Input: part model. Units: mm. Frame: model coordinates. A direction names the side the tool comes from. Coordinates: 2 decimals unless noted, no trailing zeros. Order: outer loops, then holes, each group sorted by start corner. A loop starts at its lowest first (then second) coordinate and runs counter-clockwise, first axis right, second up. Notation, with made-up numbers: (-38, 56) -> (6, 56) arc R22 cw to (6, 85) -> close; hole circle Ø10 at (3, 84.25). An arc over 180 degrees is marked (long way). One line per question, with ' | ' between items.
Autodesk Inventor part; units mm, degrees
ref_plane "YZ Plane" through (0, 0, 0) normal (1, 0, 0) x (0, 1, 0)
ref_plane "XZ Plane" through (0, 0, 0) normal (0, 1, 0) x (-1, 0, 0)
ref_plane "XY Plane" through (0, 0, 0) normal (0, 0, 1) x (1, 0, 0)
sketch "Эскиз1" plane through (0, 0, 0) normal (0, 1, 0) x (-1, 0, 0)
  line L0 (0, 0) -> (4, 0)
  line L1 (4, 0) -> (4, -23.9397)
  line L2 (4, -23.9397) -> (0, -23.9397)
  line L3 (0, -23.9397) -> (0, 0)
  line L4 (0, -23.9397) -> (11.75, -23.9397)
  line L5 (11.75, -23.9397) -> (11.75, -19.9397)
  line L6 (11.75, -19.9397) -> (0, -19.9397)
  line L7 (0, -19.9397) -> (0, -23.9397)
  line L8 (11.75, -19.9397) -> (7.75, -19.9397)
  line L9 (7.75, -19.9397) -> (7.75, -29.9397)
  line L10 (7.75, -29.9397) -> (11.75, -29.9397)
  line L11 (11.75, -29.9397) -> (11.75, -19.9397)
  line L12 (11.75, -23.9397) -> (4, -19.9397)
  line L13 (0, -19.9397) -> (7.75, -23.9397)
  point P0 (3, -20.536)
  point P1 (0, -19.9397)
  dimension "d10" = 4
  dimension "d11" = 11.75
  dimension "d36" = 29.9397
  dimension "d55" = 10
extrude "Выдавливание1" add sketch "Эскиз1" along normal blind 5
fillet "Сопряжение2" radius 3.855 4 edges at (-4, 2.5, -19.9397) (-11.75, 2.5, -19.9397) (0, 2.5, -23.9397) (-7.75, 2.5, -23.9397)
sketch "Эскиз7" plane through (-11.75, 0, -29.9397) normal (-1, 0, 0) x (0, 0, 1)
  line L0 (0, 0) -> (0, 5)
  circle A0 centre (0, 2.5) radius 2.525
  circle A1 centre (0, 2.5) radius 3.525
  point P0 (29.9397, 0)
  point P1 (0, 4.975)
  point P2 (0, 0.025)
  dimension "d37" = 5.05
  dimension "d38" = 7.05
extrude "Выдавливание5" add sketch "Эскиз7" against normal up to surface (4 mm away) contours A0 | A1
extrude "Выдавливание8" cut sketch "Эскиз7" against normal through all contours A0
sketch "Эскиз8" plane through (-4, 0, 0) normal (-1, 0, 0) x (0, 0, 1)
  line L0 (0, 0) -> (0, 5)
  circle A0 centre (0, 2.5) radius 2.525
  circle A1 centre (0, 2.5) radius 3.525
  point P0 (0, 4.975)
  point P1 (0, 0.025)
  dimension "d41" = 5.05
  dimension "d42" = 7.05
extrude "Выдавливание6" add sketch "Эскиз8" against normal up to surface (4 mm away)
extrude "Выдавливание7" cut sketch "Эскиз8" against normal through all contours A0
sketch "Эскиз9" plane through (-4, 0, -20.0847) normal (1, 0, 0) x (0, 0, -1)
  circle A0 centre (-20.0847, 2.5) radius 2.525
  circle A1 centre (-20.0847, 2.5) radius 4.025
  arc A2 (-17.5996, 5) -> (-17.5996, 0) centre (-20.0847, 2.5) ccw
  point P0 (-20.0847, 0)
  point P1 (-20.0847, 4.975)
  point P2 (-20.0847, 0.025)
  point P3 (-19.7302, 5)
  point P4 (-19.7302, 0)
  dimension "d49" = 0.5
extrude "Выдавливание9" cut sketch "Эскиз9" along normal blind 2.25 contours A0 | A1
sketch "Эскиз10" plane through (0, 0, -16.0847) normal (-1, 0, 0) x (0, 0, 1)
  arc A0 (13.5996, 0) -> (13.5996, 5) centre (16.0847, 2.5) ccw
  circle A1 centre (16.0847, 2.5) radius 3.525
  circle A2 centre (16.0847, 2.5) radius 2.525
  point P0 (12.3578, 0)
  point P1 (12.3578, 5)
  point P2 (13.5996, 5)
  point P3 (13.5996, 0)
  point P4 (13.671, 5)
  point P5 (13.671, 0)
extrude "Выдавливание10" add sketch "Эскиз10" against normal blind 2.25
fillet "Сопряжение6" radius 2.25 1 edges at (0, 2.5, -3.525)
sketch "Эскиз11" plane through (-4, 0, -16.0847) normal (-1, 0, 0) x (0, 0, 1)
  line L0 (4.9302, 5) -> (0.9302, 5) construction
  line L1 (4.9302, 6) -> (0.9302, 6)
  line L2 (0.9302, 4) -> (4.9302, 4)
  arc A0 (4.9302, 4) -> (4.9302, 6) centre (4.9302, 5) ccw
  arc A1 (0.9302, 6) -> (0.9302, 4) centre (0.9302, 5) ccw
  line L3 (0, 5) -> (12.9302, 5)
  point P0 (16.0847, 0)
  point P1 (2.9302, 5)
  dimension "d56" = 2
  dimension "d57" = 2
  dimension "d58" = 10
extrude "Выдавливание11" cut sketch "Эскиз11" against normal blind 1.55
properties part number "Рулевая тяга"
1. Cut plane C-C, the plane x = -8.75. Return loops of the section in (y, z) (3 decimals).
Recorded:
outline: (0, -27.455) arc R3.525 ccw (long way) to (5, -27.455) -> (5, -20.036) -> (0, -20.036) -> close; hole circle Ø5.05 at (2.5, -29.94)
2. Access query for faces 1 (the face through (-2.891, 2.538, -4.025)), 2 (the face through (-3, 5, -18)), 3 (the face through (-3, 4, -13)). Directions: +Z, -Z, +X, -X, +Y, -Y. A direction counts if a zero-diameter tool reaches every point of the face in a straight line with its end or side. Return the directions, or none.
Recorded:
face 1: +Z, -X | face 2: +X, -X, +Y | face 3: -X, +Y
3. Cut plane B-B, the plane y = 2.5. Return loops of the section in (x, z) (3 decimals).
Recorded:
outline: (-11.75, -33.465) -> (-7.75, -33.465) -> (-7.75, -32.465) -> (-11.75, -32.465) -> close; (-11.75, -27.415) -> (-7.731, -27.415) arc R3.855 cw to (-3.895, -23.94) -> (-3.855, -23.94) arc R3.855 ccw to (0, -20.085) -> (0, -5.775) arc R2.25 cw to (2.25, -3.525) -> (2.25, -2.525) -> (-1.75, -2.525) -> (-1.75, -4.025) -> (-4, -4.025) -> (-4, -16.085) arc R3.855 cw to (-7.855, -19.94) -> (-7.895, -19.94) arc R3.855 ccw to (-11.75, -23.795) -> close; (-1.75, 2.525) -> (2.25, 2.525) -> (2.25, 3.525) -> (-1.75, 3.525) -> close
4. Pin query (flat end, axial travel): pin 1 Ø3 at (x, y) = (-0.5, 4) entering from +Z (3 decimals); pin 2 Ø1.1 at (y, z) = (4.5, -13.5) entering from -X; pin 3 Ø3 at (x, y) = (-1.5, 2) entering from -Z; pin 4 Ø1.5 at (y, z) = (3, -14.5) entering from +X. Return the tip coordinate at first contact, or that it passes through.
Recorded:
pin 1: stops at z = 3.525 | pin 2: stops at x = -4 | pin 3: stops at z = -23.84 | pin 4: stops at x = 0
5. Cut plane A-A, the plane z = 0. Return loops of the section in (x, y) (3 decimals).
Recorded:
outline: (-1.75, -1.025) -> (2.25, -1.025) -> (2.25, -0.025) -> (-1.75, -0.025) -> close; (-1.75, 5.025) -> (2.25, 5.025) -> (2.25, 6.025) -> (-1.75, 6.025) -> close
6. Mould query, pull axis Z, two halves, no side actions, for faces 4 (the face through (-3.24, 4.3, -15.87)), 5 (the face through (-11.75, 2, -27)), 6 (the face through (-5.1, 2.54, -18.78)). Classes: released by +Z, released by -Z, zero draft, split by the parting line, or undercut.
Recorded:
face 4: undercut | face 5: zero draft | face 6: released by +Z
7. Ray query, line 1 (Y direction, x = -2, z = -19); line 2 (Z direction, x = -9.85, y = 2.5); line 3 (Y direction, x = -0.5, z = 0) (3 decimals). Return the intervals inside material, ascending. Write a range as [from, to].
Recorded:
line 1: y = [0, 5] | line 2: z = [-33.46, -32.46], [-27.41, -20.47] | line 3: y = [-1.025, -0.025], [5.025, 6.025]
8. Cut plane D-D, the plane z = -29. Return loops of the section in (x, y), and give its area (3 significant figures).
Recorded:
outline: (-11.75, -0.9) -> (-7.75, -0.9) -> (-7.75, 0.16) -> (-11.75, 0.16) -> close; (-11.75, 4.84) -> (-7.75, 4.84) -> (-7.75, 5.9) -> (-11.75, 5.9) -> close | area: 8.43 mm^2
